```python
from build123d import *

# Parameters (mm, degrees)
F1_DEPTH = 3.175


with BuildPart() as f1:
    # F0 (on Right) → F1 (new body)
    with BuildSketch(Plane.YZ):
        with BuildLine():
            Line((-40.4511333859, 29.1073653109), (-36.3753204967, 26.6437996954))
            ThreePointArc((-36.3753204967, 26.6437996954), (-35.6929146046, 28.2235683845), (-35.4597376823, 29.9285538495))
            ThreePointArc((-35.4597376823, 29.9285538495), (-35.506060347, 30.6941595257), (-35.6443525017, 31.4485951564))
            Line((-35.6443525017, 31.4485951564), (-40.2683913872, 30.3085641762))
            ThreePointArc((-40.2683913872, 30.3085641762), (-40.2338183485, 30.1199552685), (-40.2222376823, 29.9285538495))
            ThreePointArc((-40.2222376823, 29.9285538495), (-40.2805319129, 29.5023074832), (-40.4511333859, 29.1073653109))
        make_face()
        with BuildLine():
            ThreePointArc((-40.2896963754, 23.7631686688), (-38.0460118676, 24.8141752957), (-36.3753204967, 26.6437996954))
            Line((-36.3753204967, 26.6437996954), (-40.4511333859, 29.1073653109))
            ThreePointArc((-40.4511333859, 29.1073653109), (-40.8688062286, 28.649959211), (-41.4297273556, 28.3872075543))
            Line((-41.4297273556, 28.3872075543), (-40.2896963754, 23.7631686688))
        make_face()
        with BuildLine():
            ThreePointArc((-35.4597376823, 29.9285538495), (-35.6929146046, 28.2235683845), (-36.3753204967, 26.6437996954))
            Line((-36.3753204967, 26.6437996954), (-25.5064861254, 20.0742913873))
            ThreePointArc((-25.5064861254, 20.0742913873), (-23.4592684491, 24.8135974547), (-22.7597376823, 29.9285538495))
            ThreePointArc((-22.7597376823, 29.9285538495), (-22.8987056762, 32.2253708783), (-23.3135821405, 34.4886777702))
            Line((-23.3135821405, 34.4886777702), (-35.6443525017, 31.4485951564))
            ThreePointArc((-35.6443525017, 31.4485951564), (-35.506060347, 30.6941595257), (-35.4597376823, 29.9285538495))
        make_face()
        with BuildLine():
            Line((-37.2496137616, 11.4323983076), (-40.2896963754, 23.7631686688))
            ThreePointArc((-40.2896963754, 23.7631686688), (-42.7647933931, 23.6507860464), (-45.0944918364, 24.4941366638))
            Line((-45.0944918364, 24.4941366638), (-51.6640001445, 13.6253022926))
            ThreePointArc((-51.6640001445, 13.6253022926), (-44.6749048146, 11.0952504402), (-37.2496137616, 11.4323983076))
        make_face()
        with BuildLine():
            ThreePointArc((-45.0944918364, 24.4941366638), (-42.7647933931, 23.6507860464), (-40.2896963754, 23.7631686688))
            Line((-40.2896963754, 23.7631686688), (-41.4297273556, 28.3872075543))
            ThreePointArc((-41.4297273556, 28.3872075543), (-42.04850161, 28.3591118987), (-42.6309262209, 28.5699495531))
            Line((-42.6309262209, 28.5699495531), (-45.0944918364, 24.4941366638))
        make_face()
        with BuildLine():
            ThreePointArc((-22.7597376823, 29.9285538495), (-23.4592684491, 24.8135974547), (-25.5064861254, 20.0742913873))
            Line((-25.5064861254, 20.0742913873), (-20.0720689398, 16.7895372333))
            ThreePointArc((-20.0720689398, 16.7895372333), (-17.3424453714, 23.1086119897), (-16.4097376823, 29.9285538495))
            ThreePointArc((-16.4097376823, 29.9285538495), (-16.5950283409, 32.9909765546), (-17.1481969599, 36.0087190771))
            Line((-17.1481969599, 36.0087190771), (-23.3135821405, 34.4886777702))
            ThreePointArc((-23.3135821405, 34.4886777702), (-22.8987056762, 32.2253708783), (-22.7597376823, 29.9285538495))
        make_face()
        with BuildLine():
            Line((-20.0720689398, 16.7895372333), (-25.5064861254, 20.0742913873))
            ThreePointArc((-25.5064861254, 20.0742913873), (-30.518560238, 14.5854181882), (-37.2496137616, 11.4323983076))
            Line((-37.2496137616, 11.4323983076), (-35.7295724547, 5.267013127))
            ThreePointArc((-35.7295724547, 5.267013127), (-26.7548344232, 9.4710396345), (-20.0720689398, 16.7895372333))
        make_face()
        with BuildLine():
            Line((-40.2683913872, 30.3085641762), (-35.6443525017, 31.4485951564))
            ThreePointArc((-35.6443525017, 31.4485951564), (-36.6953591286, 33.6922796642), (-38.5249835283, 35.3629710351))
            Line((-38.5249835283, 35.3629710351), (-40.9885491438, 31.2871581459))
            ThreePointArc((-40.9885491438, 31.2871581459), (-40.5311430439, 30.8694853032), (-40.2683913872, 30.3085641762))
        make_face()
        with BuildLine():
            ThreePointArc((-47.975122863, 28.4085125426), (-46.9241162361, 26.1648280347), (-45.0944918364, 24.4941366638))
            Line((-45.0944918364, 24.4941366638), (-42.6309262209, 28.5699495531))
            ThreePointArc((-42.6309262209, 28.5699495531), (-43.0883323208, 28.9876223958), (-43.3510839775, 29.5485435227))
            Line((-43.3510839775, 29.5485435227), (-47.975122863, 28.4085125426))
        make_face()
        with BuildLine():
            Line((-35.7295724547, 5.267013127), (-37.2496137616, 11.4323983076))
            ThreePointArc((-37.2496137616, 11.4323983076), (-44.6749048146, 11.0952504402), (-51.6640001445, 13.6253022926))
            Line((-51.6640001445, 13.6253022926), (-54.9487542985, 8.1908851069))
            ThreePointArc((-54.9487542985, 8.1908851069), (-45.6299605253, 4.8174826371), (-35.7295724547, 5.267013127))
        make_face()
        with BuildLine():
            Line((-40.9885491438, 31.2871581459), (-38.5249835283, 35.3629710351))
            ThreePointArc((-38.5249835283, 35.3629710351), (-40.8546819716, 36.2063216525), (-43.3297789892, 36.0939390301))
            Line((-43.3297789892, 36.0939390301), (-42.1897480091, 31.4699001446))
            ThreePointArc((-42.1897480091, 31.4699001446), (-41.5709737547, 31.4979958002), (-40.9885491438, 31.2871581459))
        make_face()
        with BuildLine():
            ThreePointArc((-43.3297789892, 36.0939390301), (-40.8546819716, 36.2063216525), (-38.5249835283, 35.3629710351))
            Line((-38.5249835283, 35.3629710351), (-31.9554752202, 46.2318054064))
            ThreePointArc((-31.9554752202, 46.2318054064), (-38.9445705501, 48.7618572587), (-46.3698616031, 48.4247093913))
            Line((-46.3698616031, 48.4247093913), (-43.3297789892, 36.0939390301))
        make_face()
        with BuildLine():
            ThreePointArc((-31.9554752202, 46.2318054064), (-26.4666020211, 41.2197312938), (-23.3135821405, 34.4886777702))
            Line((-23.3135821405, 34.4886777702), (-17.1481969599, 36.0087190771))
            ThreePointArc((-17.1481969599, 36.0087190771), (-21.3522234673, 44.9834571086), (-28.6707210662, 51.666222592))
            Line((-28.6707210662, 51.666222592), (-31.9554752202, 46.2318054064))
        make_face()
        with BuildLine():
            Line((-60.3058932242, 25.3684299287), (-47.975122863, 28.4085125426))
            ThreePointArc((-47.975122863, 28.4085125426), (-48.0875054854, 30.8836095602), (-47.244154868, 33.2133080035))
            Line((-47.244154868, 33.2133080035), (-58.1129892392, 39.7828163116))
            ThreePointArc((-58.1129892392, 39.7828163116), (-60.6430410916, 32.7937209817), (-60.3058932242, 25.3684299287))
        make_face()
        with BuildLine():
            ThreePointArc((-47.244154868, 33.2133080035), (-48.0875054854, 30.8836095602), (-47.975122863, 28.4085125426))
            Line((-47.975122863, 28.4085125426), (-43.3510839775, 29.5485435227))
            ThreePointArc((-43.3510839775, 29.5485435227), (-43.3791796331, 30.1673177771), (-43.1683419788, 30.749742388))
            Line((-43.1683419788, 30.749742388), (-47.244154868, 33.2133080035))
        make_face()
        with BuildLine():
            Line((-54.9487542985, 8.1908851069), (-51.6640001445, 13.6253022926))
            ThreePointArc((-51.6640001445, 13.6253022926), (-57.1528733436, 18.6373764051), (-60.3058932242, 25.3684299287))
            Line((-60.3058932242, 25.3684299287), (-66.4712784048, 23.8483886218))
            ThreePointArc((-66.4712784048, 23.8483886218), (-62.2672518974, 14.8736505903), (-54.9487542985, 8.1908851069))
        make_face()
        with BuildLine():
            Line((-47.244154868, 33.2133080035), (-43.1683419788, 30.749742388))
            ThreePointArc((-43.1683419788, 30.749742388), (-42.750669136, 31.2071484879), (-42.1897480091, 31.4699001446))
            Line((-42.1897480091, 31.4699001446), (-43.3297789892, 36.0939390301))
            ThreePointArc((-43.3297789892, 36.0939390301), (-45.5734634971, 35.0429324032), (-47.244154868, 33.2133080035))
        make_face()
        with BuildLine():
            ThreePointArc((-46.3698616031, 48.4247093913), (-38.9445705501, 48.7618572587), (-31.9554752202, 46.2318054064))
            Line((-31.9554752202, 46.2318054064), (-28.6707210662, 51.666222592))
            ThreePointArc((-28.6707210662, 51.666222592), (-37.9895148394, 55.0396250618), (-47.88990291, 54.5900945719))
            Line((-47.88990291, 54.5900945719), (-46.3698616031, 48.4247093913))
        make_face()
        with BuildLine():
            Line((-66.4712784048, 23.8483886218), (-60.3058932242, 25.3684299287))
            ThreePointArc((-60.3058932242, 25.3684299287), (-60.6430410916, 32.7937209817), (-58.1129892392, 39.7828163116))
            Line((-58.1129892392, 39.7828163116), (-63.5474064249, 43.0675704656))
            ThreePointArc((-63.5474064249, 43.0675704656), (-66.9208088947, 33.7487766925), (-66.4712784048, 23.8483886218))
        make_face()
        with BuildLine():
            ThreePointArc((-58.1129892392, 39.7828163116), (-53.1009151267, 45.2716895107), (-46.3698616031, 48.4247093913))
            Line((-46.3698616031, 48.4247093913), (-47.88990291, 54.5900945719))
            ThreePointArc((-47.88990291, 54.5900945719), (-56.8646409415, 50.3860680645), (-63.5474064249, 43.0675704656))
            Line((-63.5474064249, 43.0675704656), (-58.1129892392, 39.7828163116))
        make_face()
    extrude(amount=F1_DEPTH)


solid = f1.part
```
Check sheet for the modelled part. Datum: model origin and axes. Units: mm. A direction names the side the tool comes from. Give positions to 0.01 mm unless a question says otherwise; leave off trailing zeros. Write each loop counter-clockwise with the first axis right and the second up, starting at its lowest first coordinate (ties: lowest second). Pieces come first, ordered by that corner, then holes. Notation, with made-up numbers: (79.25, 80) - (117.25, 80) arc R32 ccw to (117.25, 117) - close; hole circle Ø5 at (52.5, 37). An arc over 180 degrees is marked (long way). Answer as a JSON object with one key per item and string values. Group by question number.
1) Thickness scan on probe 1 along Y at (x, z) = (2, 29.5); probe 2 along Y at (x, z) = (2.1, 17); probe 3 along Z at (x, y) = (0.7, -57). Record the ranges inside material, lowest first. Write a range as from..to.
2) Depth check by flat-ended pin: P1, Ø6, axis at y = -39, z = 11, coming from the -X side. Enter the tip coordinate at first touch or a pass-through.
3) Sectioned sample at D-D (y = -44). Record the cut outline in (x, z) (3 decimals), then the cut area to 3 significant figures.
4) Release check for a two-part mould opening along Z. For faces 3 (the face through (1.565, -38.074, 24.794)), 4 (the face through (3.175, -42, 25)) record: pulls with the +Z half, pulls with the -Z half, needs draft (parallel to the pull), parting line crosses it, or undercut.
5) Access from +Z, -Z, +X, -X, +Y, -Y to the whole of each face (thin tool, end or side, straight path). Record for faces 1 (the face through (1.565, -31.017, 23.405)), 2 (the face through (0, -42, 25)).
6) Sectioned sample at A-A (x = 1.3). Give the number of separate pieces and of enclosed holes in the cut face, then the cut area to 3 significant figures.
7) Sectioned sample at B-B (y = -50.5). Record the cut outline in (x, z) (3 decimals), then the cut area to 3 significant figures.
8) Sectioned sample at C-C (z = 19). Record the cut outline in (x, y) (3 decimals), then the cut area to 3 significant figures.
Geometry results:
{
 "1": {"probe 1": "y = -67.21..-43.34, -40.28..-16.41", "probe 2": "y = -63.67..-55.8, -49.62..-38.62, -27.82..-19.95", "probe 3": "z = 9.57..18.43, 26.18..39.11, 41.42..50.29"},
 "2": {"P1": "stops at x = 0"},
 "3": {"outline": "(0, 4.623) - (3.175, 4.623) - (3.175, 35.889) - (0, 35.889) - close; (0, 38.812) - (3.175, 38.812) - (3.175, 55.234) - (0, 55.234) - close", "area": "151 mm^2"},
 "4": {"face 3": "undercut", "face 4": "needs draft"},
 "5": {"face 1": "+X, -X", "face 2": "+Z, -Z, -X, +Y, -Y"},
 "6": {"separate pieces": "1", "enclosed holes": "5", "area": "1,510 mm^2"},
 "7": {"outline": "(0, 6.061) - (3.175, 6.061) - (3.175, 15.551) - (0, 15.551) - close; (0, 27.786) - (3.175, 27.786) - (3.175, 35.181) - (0, 35.181) - close; (0, 46.881) - (3.175, 46.881) - (3.175, 53.796) - (0, 53.796) - close", "area": "75.6 mm^2"},
 "8": {"outline": "(0, -64.738) - (3.175, -64.738) - (3.175, -57.413) - (0, -57.413) - close; (0, -48.415) - (3.175, -48.415) - (3.175, -39.115) - (0, -39.115) - close; (0, -26.206) - (3.175, -26.206) - (3.175, -18.881) - (0, -18.881) - close", "area": "76.0 mm^2"}
}
